Geometry check sheet. Reference: the model listing, model coordinates, mm. Face numbers are marked on the shaded views. Give positions to 0.01 mm unless a question says otherwise; leave off trailing zeros. Loops run counter-clockwise (first coordinate to the right, second up) from the corner with the lowest first, then second, coordinate; pieces in that order, holes last. Notation, with made-up numbers: (70, 47.5) -> (87, 47.5) arc R20 cw to (87, 76.5) -> close; hole circle Ø3 at (-35, -11.5). An arc over 180 degrees is marked (long way). Write each question's results on one line, items separated by ' | '. Start each with the question number.
1) Sectioned sample at A-A on z = 85.5. Record the cut outline in (x, y), then the cut area to 3 significant figures.
2) Scan lines: line 1 (Y direction, x = -2, z = 83); line 2 (Z direction, x = -7.25, y = -20.5); line 3 (Z direction, x = -9, y = -22.5). Record each from-to range of solid material in increasing order. Write a range as from..to.
3) Sectioned sample at B-B on x = -9.5. Record the cut outline in (y, z), then the cut area to 3 significant figures.
4) Depth check by flat-ended pin: pin 1 (12 mm diameter, centred on x = -9, z = 64, fed in from -Y); pin 2 (4 mm diameter, centred on y = 2.5, z = 82, fed in from -X); pin 3 (1 mm diameter, centred on x = 0.5, y = 0.5, fed in from +Z). Enter the tip coordinate at first touch or a pass-through.
5) Sectioned sample at D-D on z = 61. Record the cut outline in (x, y) (3 decimals).
6) Draft check along Z on the marked faces 1, 2, 3 and 4. Enter one of: pulls with the +Z half, pulls with the -Z half, needs draft (parallel to the pull), parting line crosses it, or undercut.
7) Sectioned sample at C-C on y = 9.5. Record the cut outline in (x, z), then the cut area to 3 significant figures.
```python
from build123d import *

# Parameters (mm, degrees)
SKETCH002_R  = 13.975
PAD002_DEPTH = 15
SKETCH003_R  = 15
PAD003_DEPTH = 25
SKETCH004_R  = 3
PAD004_DEPTH = 15
BOX_W        = 44
BOX_H        = 61
BOX_DEPTH    = 44


with BuildPart() as part:
    # Sketch002 (on DatumPlane) → Pad002 (new body)
    with BuildSketch(Plane.XY.offset(73)):
        Circle(SKETCH002_R)
    extrude(amount=-PAD002_DEPTH)

    # Sketch003 (on DatumPlane) → Pad003 (join)
    with BuildSketch(Plane.XY.offset(73)):
        Circle(SKETCH003_R)
    extrude(amount=PAD003_DEPTH)

    # Sketch004 (on DatumPlane) → Pad004 (join, symmetric)
    with BuildSketch(Plane(origin=(0, 0, 85.5), x_dir=(0, 0, -1), z_dir=(1, 0, 0))):
        with BuildLine():
            ThreePointArc((-6.5469509024, -19.0812783951), (-2.6386229499, -29.760680346), (7.3361760867, -24.2991752795))
            Line((7.3361760867, -24.2991752795), (12.5, 0))
            Line((4.1169733945, 0), (12.5, 0))
            Line((-6.5469509024, -19.0812783951), (4.1169733945, 0))
        make_face()
        with Locations((0, -22.7401626351)):
            Circle(SKETCH004_R, mode=Mode.SUBTRACT)
    extrude(amount=PAD004_DEPTH, both=True)

    # Box → Box (cut)
    with BuildSketch(Plane(origin=(-23, -30.474162324, 98.414074175), x_dir=(1, 0, 0), z_dir=(0, 0.487851232, 0.872926787))):
        with Locations((22, 30.5)):
            Rectangle(BOX_W, BOX_H)
    extrude(amount=BOX_DEPTH, mode=Mode.SUBTRACT)


solid = part.part
```
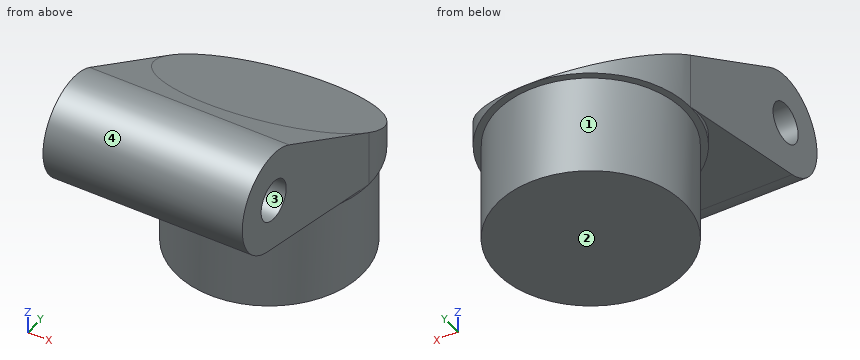
Result:
1) outline: (-15, -30.24) -> (15, -30.24) -> (15, -25.74) -> (-15, -25.74) -> close; (-15, -19.74) -> (15, -19.74) -> (15, -7.37) -> (-15, -7.37) -> close | area: 506 mm^2
2) line 1: -29.81..-24.4, -21.08..-2.89 | line 2: 77.36..83.5, 87.5..92.66 | line 3: 77.78..82.51, 88.49..93
3) outline: (-24.3, 78.16) -> (-11.61, 75.47) -> (-11.61, 73) -> (-10.25, 73) -> (-10.25, 58) -> (10.25, 58) -> (10.25, 73) -> (11.61, 73) -> (11.61, 74.9) -> (-19.08, 92.05) arc R7.5 ccw (long way) to start; hole circle Ø6 at (-22.74, 85.5) | area: 720 mm^2
4) pin 1: y = -13.65 | pin 2: x = -14.98 | pin 3: z = 81.38
5) outline: circle Ø27.95 at (0, 0)
6) face 1: needs draft | face 2: pulls with the -Z half | face 3: undercut | face 4: parting line crosses it
7) outline: (-11.61, 73) -> (-10.25, 73) -> (-10.25, 58) -> (10.25, 58) -> (10.25, 73) -> (11.61, 73) -> (11.61, 76.07) -> (-11.61, 76.07) -> close | area: 379 mm^2
